Input: part model. Units: mm. Frame: model coordinates. Face numbers are marked on the shaded views. A direction names the side the tool comes from. Coordinates: 2 decimals unless noted, no trailing zeros. Write each loop counter-clockwise with the first axis right and the second up, starting at its lowest first coordinate (ties: lowest second). Pieces come first, ordered by that corner, then holes. Notation, with made-up numbers: (-32.5, 71.25) - (26.5, 71.25) arc R13 cw to (26.5, 85.25) - close; hole circle Ø8 at (9, -29.75). An arc over 180 degrees is marked (long way). Use a Markdown table: item, result. Add a question column.
Q1. Material intervals for probe 1 along Z at (x, y) = (-33, -1.2); probe 2 along X at (y, z) = (22.5, 1); probe 3 along Y at (x, z) = (47, 18), sorted ascending. Write a range as from..to.
Q2. Section query B-B (z = 15). Return the cut outline in (x, y), then the cut area to 3 significant figures.
Q3. Section query D-D (z = 9.75). Return the cut outline in (x, y), then the cut area to 3 significant figures.
Q4. Pin query (flat end, axial travel): P1, Ø2.5, axis at x = 45, z = 15, coming from the +Y side; P2, Ø4, axis at y = 45, z = 9, coming from the +X side; P3, Ø1.5, axis at x = 6, z = 12.5, coming from the +Y side; P4, Ø1, axis at x = -29.5, z = 7, coming from the +Y side. Return the tip coordinate at first contact, or that it passes through.
Q5. Section query C-C (x = -33). Return the cut outline in (y, z), then the cut area to 3 significant figures.
Q6. Mould query, pull axis X, two halves, no side actions, for the marked faces 5, 6 and 7. Classes: released by +X, released by -X, zero draft, split by the parting line, or undercut.
Q7. Section query A-A (y = 7). Return the cut outline in (x, z).
Q8. Set-up query: the marked faces 1, 2, 3 and 4. Return all of +Z, -Z, +X, -X, +Y, -Y with unobstructed straight access to the full face (end or side cutting, diameter ignored); none if empty.
from build123d import *

# Parameters (mm, degrees)
BOSS_EXTRUDE1_DEPTH = 20
SKETCH2_R           = 2
CUT_EXTRUDE1_DEPTH  = 81.324342512


with BuildPart() as part:
    # Sketch1 → Boss-Extrude1 (new body)
    with BuildSketch(Plane.XY):
        with BuildLine():
            Line((-18, 0), (-18, 30))
            ThreePointArc((-18, 30), (6, 54), (30, 30))
            Line((30, 30), (30, 0))
            Line((30, 0), (56, 0))
            Line((56, 0), (56, -2))
            Line((56, -2), (26, -2))
            Line((26, -2), (26, 0))
            Line((26, 0), (26, 30))
            ThreePointArc((26, 30), (6, 50), (-14, 30))
            Line((-14, 30), (-14, 0))
            Line((-14, 0), (-14, -2))
            Line((-14, -2), (-44, -2))
            Line((-44, -2), (-44, 0))
            Line((-44, 0), (-18, 0))
        make_face()
    extrude(amount=BOSS_EXTRUDE1_DEPTH)

    # Sketch2 → Cut-Extrude1 (cut, through all)
    with BuildSketch(Plane(origin=(0, 0, 0), x_dir=(1, 0, 0), z_dir=(0, 1, 0))):
        with Locations(Location((-33, -5, 0), (0, 0, 180))):
            Circle(SKETCH2_R)
        with Locations(Location((-33, -15, 0), (0, 0, 180))):
            Circle(SKETCH2_R)
        with Locations(Location((45, -5, 0), (0, 0, 180))):
            Circle(SKETCH2_R)
        with Locations((45, -15)):
            Circle(SKETCH2_R)
    extrude(amount=-CUT_EXTRUDE1_DEPTH, mode=Mode.SUBTRACT)


solid = part.part
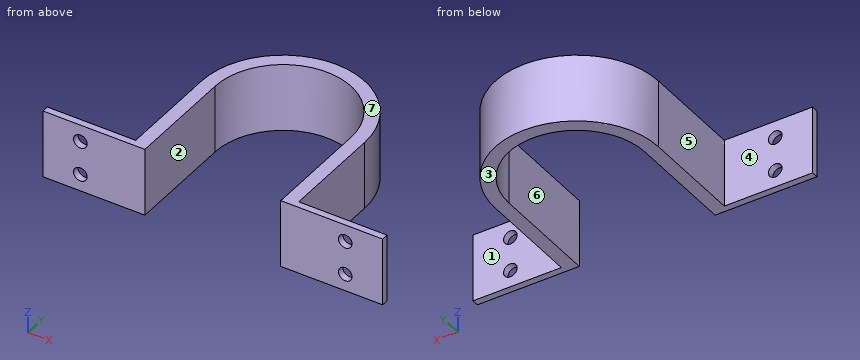
Values follow:
| question | item | result |
|---|---|---|
| 1 | probe 1 | 0..3, 7..13, 17..20 |
| 1 | probe 2 | -18..-14, 26..30 |
| 1 | probe 3 | -2..0 |
| 2 | outline | (-44, -2) - (-35, -2) - (-35, 0) - (-44, 0) - close; (-31, -2) - (-14, -2) - (-14, 30) arc R20 cw to (26, 30) - (26, -2) - (43, -2) - (43, 0) - (30, 0) - (30, 30) arc R24 ccw to (-18, 30) - (-18, 0) - (-31, 0) - close; (47, -2) - (56, -2) - (56, 0) - (47, 0) - close |
| 2 | area | 620 mm2 |
| 3 | outline | (-44, -2) - (-14, -2) - (-14, 30) arc R20 cw to (26, 30) - (26, -2) - (56, -2) - (56, 0) - (30, 0) - (30, 30) arc R24 ccw to (-18, 30) - (-18, 0) - (-44, 0) - close |
| 3 | area | 636 mm2 |
| 4 | P1 | through |
| 4 | P2 | x = 26.17 |
| 4 | P3 | y = 54 |
| 4 | P4 | y = 0 |
| 5 | outline | (-2, 0) - (0, 0) - (0, 3) - (-2, 3) - close; (-2, 7) - (0, 7) - (0, 13) - (-2, 13) - close; (-2, 17) - (0, 17) - (0, 20) - (-2, 20) - close |
| 5 | area | 24.0 mm2 |
| 6 | face 5 | released by -X |
| 6 | face 6 | undercut |
| 6 | face 7 | zero draft |
| 7 | outline | (-18, 0) - (-14, 0) - (-14, 20) - (-18, 20) - close; (26, 0) - (30, 0) - (30, 20) - (26, 20) - close |
| 8 | face 1 | +Z, -Z, +X, +Y |
| 8 | face 2 | +Z, -Z, -Y |
| 8 | face 3 | -Z, +X, -X, +Y, -Y |
| 8 | face 4 | +Z, -Z, -X, +Y |
